from build123d import *

# Parameters (mm, degrees)
PAD_DEPTH     = 5
SKETCH001_R   = 13.875
SKETCH001_R_2 = 6.4
SKETCH001_R_3 = 4.55
PAD001_DEPTH  = 2


with BuildPart() as part:
    # Sketch → Pad (new body)
    with BuildSketch(Plane.XY):
        with BuildLine():
            ThreePointArc((45.653278, -37.879963), (0, -26.25), (-45.653278, -37.879963))
            ThreePointArc((-79.129462, -1.094945), (-76.833677, -32.630667), (-45.653278, -37.879963))
            ThreePointArc((79.129462, -1.094945), (0, 41), (-79.129462, -1.094945))
            ThreePointArc((45.653278, -37.879963), (76.833677, -32.630667), (79.129462, -1.094945))
        make_face()
    extrude(amount=PAD_DEPTH)

    # Sketch001 (on Face6 of Pad) → Pad001 (join)
    with BuildSketch(Plane.XY.offset(5)):
        with Locations((-45.704856, -2.533086)):
            Circle(SKETCH001_R)
        with Locations((30.286027, -14.783871)):
            Circle(SKETCH001_R_2)
        with Locations((43.390221, -5.090053)):
            Circle(SKETCH001_R_2)
        with Locations((59.680872, -4.538045)):
            Circle(SKETCH001_R_2)
        with Locations((19.747467, 2.384254)):
            Circle(SKETCH001_R_3)
        with Locations((32.104855, 10.886898)):
            Circle(SKETCH001_R_3)
        with Locations((46.728688, 14.225088)):
            Circle(SKETCH001_R_3)
    extrude(amount=PAD001_DEPTH)


solid = part.part
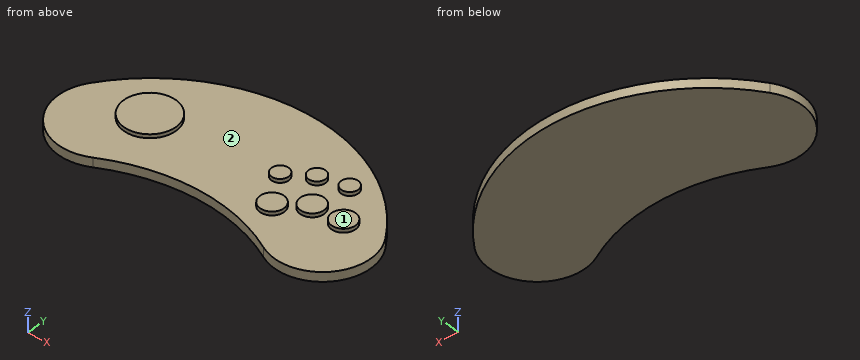
Design review of the part built by this model. Coordinates are the model's own, in mm. Face numbers are marked on the shaded views. Round coordinates to 2 decimals unless told otherwise and drop trailing zeros. Write each loop counter-clockwise with the first axis right and the second up, starting at its lowest first coordinate (ties: lowest second). Pieces come first, ordered by that corner, then holes.
Item 1: Consider section C-C on x = -30. Give the boundary of the cut face in (y, z), and give its area (3 significant figures).
Item 2: Draft analysis for pull direction X (two halves, no side actions). For the marked faces 1 and 2, state which applies: released by +X, released by -X, zero draft, split by the parting line, or undercut.
Item 3: For pin 1 Ø1.5 at (y, z) = (0, 6.5) entering from -X; pin 2 Ø1 at (y, z) = (-25.5, 6) entering from -X; pin 3 Ø12 at (x, y) = (49, -30.5) entering from +Z; pin 4 Ø4 at (x, z) = (-51.5, 3.5) entering from +Y, all flat-tipped, find the tip position at first contact; note any pin that passes through.
Item 4: Consider section A-A on y = -29.5. Give the boundary of the cut face in (x, z).
Item 5: Wall thickness on L1, parallel to Z at x = -55.5, y = -18; L2, parallel to Y at x = 35.5, z = 5.5; L3, parallel to Y at x = 2.5, z = 2.5: over which ranges is each line inside the solid? List them lowest first.
Item 6: Consider section B-B on z = 3. Give the boundary of the cut face in (x, y), and give its area (4 significant figures).
Check values:
1. outline: (-31.09, 0) - (36.16, 0) - (36.16, 5) - (-31.09, 5) - close
1. area: 336 mm2
2. face 1: zero draft
2. face 2: undercut
3. pin 1: stops at x = -59.46
3. pin 2: passes through
3. pin 3: stops at z = 5
3. pin 4: stops at y = 27.16
4. outline: (-79.27, 0) - (-24.69, 0) - (-24.69, 5) - (-79.27, 5) - close; (24.69, 0) - (79.27, 0) - (79.27, 5) - (24.69, 5) - close
5. L1: z = 0 to 5
5. L2: y = -18.5 to -11.07, 7.86 to 13.92
5. L3: y = -26.28 to 40.97
6. outline: (-79.13, -1.09) arc R25.6 ccw to (-45.65, -37.88) arc R95.42 cw to (45.65, -37.88) arc R25.6 ccw to (79.13, -1.09) arc R95.42 ccw to start
6. area: 10,000 mm2
